Source: CAD feature listing. Evaluate the final solid. Frame: model axes, mm. A direction names the side the tool comes from. Coordinates: 2 decimals unless noted, no trailing zeros. Loops run counter-clockwise (first coordinate to the right, second up) from the corner with the lowest first, then second, coordinate; pieces in that order, holes last.
from build123d import *
from build123d.topology import SkipClean

# Parameters (mm, degrees)
BOSS_EXTRU_1_DEPTH                   = 4
BOSS_EXTRU_6_DEPTH                   = 3
ENL_V_MAT_EXTRU_9_DEPTH              = 1.5
ESQUISSE18_W                         = 26
ESQUISSE18_H                         = 4
BOSS_EXTRU_5_DEPTH                   = 3.5
ESQUISSE24_W                         = 26
ESQUISSE24_H                         = 9
ESQUISSE24_R                         = 1.6
BOSS_EXTRU_7_DEPTH                   = 0.3
ESQUISSE25_W                         = 26
ESQUISSE25_H                         = 12
BOSS_EXTRU_8_DEPTH                   = 3
ENL_V_MAT_EXTRU_13_REACH             = 155.177
ENL_V_MAT_EXTRU_13_DIRECTION_2_REACH = 155.177
ENL_V_MAT_EXTRU_14_REACH             = 155.177
ENL_V_MAT_EXTRU_14_DIRECTION_2_REACH = 155.177
ENL_V_MAT_EXTRU_15_REACH             = 161.061
ESQUISSE38_W                         = 26
ESQUISSE38_H                         = 10.68641461
ESQUISSE38_R                         = 1.6
BOSS_EXTRU_10_DEPTH                  = 0.09


# Read off the part's stored shape, not the designer's step: Fraisage pour vis à tête fraisée à 6 pans creux M31
with BuildPart() as part:
    # Esquisse1 → Boss.-Extru.1 (new body)
    with BuildSketch(Plane(origin=(0, 0, 0), x_dir=(1, 0, 0), z_dir=(0, 1, 0))):
        with BuildLine():
            Line((-13, -130), (-13, -76))
            ThreePointArc((-13, -76), (-17.360668588, -59.081626241), (-29.356078322, -46.378990826))
            Line((-29.356078322, -46.378990826), (-75, -17.65))
            Line((-75, -17.65), (-75, 0))
            Line((-75, 0), (75, 0))
            Line((75, 0), (75, -17.65))
            Line((75, -17.65), (29.356078322, -46.378990826))
            ThreePointArc((29.356078322, -46.378990826), (17.360668588, -59.081626241), (13, -76))
            Line((13, -76), (13, -130))
            Line((13, -130), (-13, -130))
        make_face()
    extrude(amount=BOSS_EXTRU_1_DEPTH)

    # Esquisse21 → Boss.-Extru.6 (add)
    with BuildSketch(Plane(origin=(0, 0, 0), x_dir=(-1, 0, 0), z_dir=(0, -1, 0))):
        Polygon((75, 0), (69, 0), (69, -21.426492874), (75, -17.65), align=None)
        Polygon((-75, 0), (-69, 0), (-69, -21.426492874), (-75, -17.65), align=None)
    extrude(amount=BOSS_EXTRU_6_DEPTH)

    # Fraisage pour vis _ t_te frais_e _ 6 2 → Fraisage pour vis à tête fraisée à 6 pans creux M31 (revolve, cut)
    with BuildSketch(Plane.XY.offset(93.29)):
        Polygon((0, 0), (1.6, 0), (1.6, 2.3), (2.9, 3.6), (2.9, 4), (0, 4), align=None)
    revolve(axis=Axis((0, 0, 93.29), (0, 1, 0)), mode=Mode.SUBTRACT)

    # Fraisage pour vis _ t_te frais_e _ 6 3 o → Fraisage pour vis _ t_te frais_e _ 6 3 (revolve, cut)
    with BuildSketch(Plane(origin=(-72, 0, 8.91), x_dir=(1, 0, 0), z_dir=(0, 0, 1))):
        Polygon((0, -3), (1.6, -3), (1.6, 2.3), (2.9, 3.6), (2.9, 4), (0, 4), align=None)
    revolve(axis=Axis((-72, 0, 8.91), (0, 1, 0)), mode=Mode.SUBTRACT)

    # Fraisage pour vis _ t_te frais_e _ 6 4 o → Fraisage pour vis _ t_te frais_e _ 6 4 (revolve, cut)
    with BuildSketch(Plane(origin=(72, 0, 8.91), x_dir=(1, 0, 0), z_dir=(0, 0, 1))):
        Polygon((0, -3), (1.6, -3), (1.6, 2.3), (2.9, 3.6), (2.9, 4), (0, 4), align=None)
    revolve(axis=Axis((72, 0, 8.91), (0, 1, 0)), mode=Mode.SUBTRACT)

    # Fraisage pour vis _ t_te frais_e _ 6 5 o → Fraisage pour vis _ t_te frais_e _ 6 5 (revolve, cut)
    with BuildSketch(Plane(origin=(19.84, 0, 13.45), x_dir=(1, 0, 0), z_dir=(0, 0, 1))):
        Polygon((0, 0), (1.6, 0), (1.6, 2.3), (2.9, 3.6), (2.9, 4), (0, 4), align=None)
    revolve(axis=Axis((19.84, 0, 13.45), (0, 1, 0)), mode=Mode.SUBTRACT)

    # Fraisage pour vis _ t_te frais_e _ 6 6 o → Fraisage pour vis _ t_te frais_e _ 6 6 (revolve, cut)
    with BuildSketch(Plane(origin=(-12.85, 0, 13.45), x_dir=(1, 0, 0), z_dir=(0, 0, 1))):
        Polygon((0, 0), (1.6, 0), (1.6, 2.3), (2.9, 3.6), (2.9, 4), (0, 4), align=None)
    revolve(axis=Axis((-12.85, 0, 13.45), (0, 1, 0)), mode=Mode.SUBTRACT)

    # Fraisage pour vis _ t_te frais_e _ 6 7 o → Fraisage pour vis _ t_te frais_e _ 6 7 (revolve, cut)
    with BuildSketch(Plane(origin=(61.15, 0, 10.45), x_dir=(1, 0, 0), z_dir=(0, 0, 1))):
        Polygon((0, 0), (1.6, 0), (1.6, 2.3), (2.9, 3.6), (2.9, 4), (0, 4), align=None)
    revolve(axis=Axis((61.15, 0, 10.45), (0, 1, 0)), mode=Mode.SUBTRACT)

    # Esquisse16 → Enlèv. mat.-Extru.9 (cut)
    with BuildSketch(Plane(origin=(0, 0, 0), x_dir=(-1, 0, 0), z_dir=(0, 0, -1))):
        Polygon((16.25, 0), (12.25, 4), (-24.5, 4), (-28.5, 0), align=None)
    extrude(amount=-ENL_V_MAT_EXTRU_9_DEPTH, mode=Mode.SUBTRACT)

    # Esquisse18 → Boss.-Extru.5 (add)
    with BuildSketch(Plane.XY.offset(130)):
        with Locations((0, 2)):
            Rectangle(ESQUISSE18_W, ESQUISSE18_H)
    extrude(amount=BOSS_EXTRU_5_DEPTH)

    # Esquisse24 → Boss.-Extru.7 (add)
    with SkipClean():  # the faces are left unmerged after this step: merging them gives an invalid solid
        with BuildSketch(Plane(origin=(0, 0, 0), x_dir=(-1, 0, 0), z_dir=(0, -1, 0))):
            with Locations((0, -93.29)):
                Rectangle(ESQUISSE24_W, ESQUISSE24_H)
            with Locations(Location((0, -93.29, 0), (0, 0, 270))):
                Circle(ESQUISSE24_R, mode=Mode.SUBTRACT)
        extrude(amount=BOSS_EXTRU_7_DEPTH)

    # Esquisse25 → Boss.-Extru.8 (add)
    with SkipClean():  # the faces are left unmerged after this step: merging them gives an invalid solid
        with BuildSketch(Plane(origin=(0, 0, 0), x_dir=(-1, 0, 0), z_dir=(0, -1, 0))):
            with Locations((0, -127.5)):
                Rectangle(ESQUISSE25_W, ESQUISSE25_H)
        extrude(amount=BOSS_EXTRU_8_DEPTH)

    # Esquisse26 → Enlèv. mat.-Extru.13 (cut, up to next)
    with BuildSketch(Plane(origin=(0, 0, 0), x_dir=(0, 0, -1), z_dir=(1, 0, 0)), mode=Mode.PRIVATE) as enl_v_mat_extru_13_sk1:
        Polygon((-121.5, -3), (-133.5, -1.738749177), (-133.5, -3), align=None)
    enl_v_mat_extru_13_tool1 = extrude(enl_v_mat_extru_13_sk1.sketch, amount=-ENL_V_MAT_EXTRU_13_REACH, mode=Mode.PRIVATE) & part.part
    add(enl_v_mat_extru_13_tool1.solids().sort_by_distance((0, -2.579583, 129.5))[0], mode=Mode.SUBTRACT)

    # Esquisse26 → Enlèv. mat.-Extru.13 direction 2 (cut, up to next)
    with BuildSketch(Plane(origin=(0, 0, 0), x_dir=(0, 0, -1), z_dir=(1, 0, 0)), mode=Mode.PRIVATE) as enl_v_mat_extru_13_direction_2_sk1:
        Polygon((-121.5, -3), (-133.5, -1.738749177), (-133.5, -3), align=None)
    enl_v_mat_extru_13_direction_2_tool1 = extrude(enl_v_mat_extru_13_direction_2_sk1.sketch, amount=ENL_V_MAT_EXTRU_13_DIRECTION_2_REACH, mode=Mode.PRIVATE) & part.part
    add(enl_v_mat_extru_13_direction_2_tool1.solids().sort_by_distance((0, -2.579583, 129.5))[0], mode=Mode.SUBTRACT)

    # Esquisse34 → Enlèv. mat.-Extru.14 (cut, up to next)
    with BuildSketch(Plane(origin=(0, 0, 0), x_dir=(0, 0, -1), z_dir=(1, 0, 0)), mode=Mode.PRIVATE) as enl_v_mat_extru_14_sk1:
        Polygon((-133.5, 4), (-131.824861428, 4), (-132.439740849, -1.850186904), (-133.5, -1.738749177), align=None)
    enl_v_mat_extru_14_tool1 = extrude(enl_v_mat_extru_14_sk1.sketch, amount=-ENL_V_MAT_EXTRU_14_REACH, mode=Mode.PRIVATE) & part.part
    add(enl_v_mat_extru_14_tool1.solids().sort_by_distance((0, 1.317192, 132.802089))[0], mode=Mode.SUBTRACT)

    # Esquisse34 → Enlèv. mat.-Extru.14 direction 2 (cut, up to next)
    with BuildSketch(Plane(origin=(0, 0, 0), x_dir=(0, 0, -1), z_dir=(1, 0, 0)), mode=Mode.PRIVATE) as enl_v_mat_extru_14_direction_2_sk1:
        Polygon((-133.5, 4), (-131.824861428, 4), (-132.439740849, -1.850186904), (-133.5, -1.738749177), align=None)
    enl_v_mat_extru_14_direction_2_tool1 = extrude(enl_v_mat_extru_14_direction_2_sk1.sketch, amount=ENL_V_MAT_EXTRU_14_DIRECTION_2_REACH, mode=Mode.PRIVATE) & part.part
    add(enl_v_mat_extru_14_direction_2_tool1.solids().sort_by_distance((0, 1.317192, 132.802089))[0], mode=Mode.SUBTRACT)

    # Esquisse33 → Enlèvement de matière-Révolution1 (revolve, cut)
    with SkipClean():  # the faces are left unmerged after this step: merging them gives an invalid solid
        with BuildSketch(Plane(origin=(8.5, 0, 0), x_dir=(0, 0, -1), z_dir=(1, 0, 0))):
            Polygon((-124.928461333, 5.421822245), (-125.766498931, -2.551572893), (-127.357733964, -2.384327351), (-126.939620111, 1.59376023), (-128.08332029, 1.713967963), (-127.885090335, 3.6), (-127.663396545, 5.709275519), align=None)
        enl_vement_de_mati_re_r_volution1 = revolve(axis=Axis((8.5, 5.421822245, 124.928461333), (0, -0.9945218953682737, 0.10452846326764909)), mode=Mode.SUBTRACT)

    # Symétrie1: Enlèvement de matière-Révolution1 across plane
    with SkipClean():  # the faces are left unmerged after this step: merging them gives an invalid solid
        add(enl_vement_de_mati_re_r_volution1.mirror(Plane(origin=(0, 0, 0), x_dir=(0, 0, 1), z_dir=(1, 0, 0))), mode=Mode.SUBTRACT)

    # Esquisse37 → Enlèv. mat.-Extru.15 (cut, up to next)
    with BuildSketch(Plane(origin=(13, 0, 0), x_dir=(0, 0, -1), z_dir=(1, 0, 0)), mode=Mode.PRIVATE) as enl_v_mat_extru_15_sk1:
        Polygon((-121.5, 0), (-121.811867536, -2.967221401), (-121.5, -3), align=None)
    enl_v_mat_extru_15_tool1 = extrude(enl_v_mat_extru_15_sk1.sketch, amount=-ENL_V_MAT_EXTRU_15_REACH, mode=Mode.PRIVATE) & part.part
    add(enl_v_mat_extru_15_tool1.solids().sort_by_distance((13, -1.989074, 121.603956))[0], mode=Mode.SUBTRACT)

    # Esquisse38 → Boss.-Extru.10 (add)
    with SkipClean():  # the faces are left unmerged after this step: merging them gives an invalid solid
        with BuildSketch(Plane(origin=(0, -15.597856618, 1.639400792), x_dir=(1, 0, 0), z_dir=(0, -0.9945218953682737, 0.10452846326765036))):
            with Locations((0, 126.177617592)):
                Rectangle(ESQUISSE38_W, ESQUISSE38_H)
            with Locations(Location((-8.5, 124.810824897, 0), (0, 0, 90))):
                Circle(ESQUISSE38_R, mode=Mode.SUBTRACT)
            with Locations(Location((8.5, 124.810824897, 0), (0, 0, 90))):
                Circle(ESQUISSE38_R, mode=Mode.SUBTRACT)
        extrude(amount=BOSS_EXTRU_10_DEPTH)


solid = part.part
Q1. Draft query along Z for faces 1 (the flat face through (-1, 0, 24)), 2 (the flat face through (-44, 2, 0)), 3 (the cylindrical face through (-0.378, 3.803, 90.415)), 4 (the flat face through (-0.18, -2.49, 127.21)). Return one class per face: +Z half, -Z half, draft (parallel to the pull), parting line (faces both ways), or undercut.
Q2. Section B-B, the plane x = -22. Return the cut outline in (y, z), plus the area to 3 significant figures.
Q3. Line query: line 1 along X through (y, z) = (2.25, 123.5); line 2 along Z through (x, y) = (0, 3.75); line 3 along X through (y, z) = (3.85, 10.45). Output: solid intervals per line, ascending.
Q4. Contact query for flat-ended pins moving along their axis: pin 1 Ø4.5 at (x, z) = (0, 93.29) entering from +Y; pin 2 Ø3.5 at (x, z) = (61.15, 10.45) entering from +Y; pin 3 Ø6.5 at (x, z) = (72.5, 7.5) entering from -Y; pin 4 Ø2.5 at (x, z) = (-12.85, 13.45) entering from +Y. Output: stop coordinate, or through.
Q5. Section A-A, the plane z = 78. Return the cut outline in (x, y), plus the area to 3 significant figures.
Q6. Access query for faces 5 (the cylindrical face through (-13.48, 3.8, 16.28)), 6 (the flat face through (13, 1, 104)), 7 (the flat face through (-13, 1, 104)). Directions: +Z, -Z, +X, -X, +Y, -Y. A direction counts if a zero-diameter tool reaches every point of the face in a straight line with its end or side. Return the directions, or none.
Derived:
1. face 1: draft
1. face 2: -Z half
1. face 3: undercut
1. face 4: +Z half
2. outline: (0, 0) - (4, 0) - (4, 52.57) - (0, 52.57) - close
2. area: 210 mm2
3. line 1: x = -13 to -10.62, -6.38 to 6.38, 10.62 to 13
3. line 2: z = 1.5 to 90.39, 96.19 to 131.85
3. line 3: x = -75 to -74.46, -69.54 to 58.25, 64.05 to 69.54, 74.46 to 75
4. pin 1: stops at y = 2.95
4. pin 2: stops at y = 2.45
4. pin 3: stops at y = -3
4. pin 4: passes through
5. outline: (-13, 0) - (13, 0) - (13, 4) - (-13, 4) - close
5. area: 104 mm2
6. face 5: +Y
6. face 6: +Z, +X, +Y, -Y
6. face 7: +Z, -X, +Y, -Y
